```python
from build123d import *

# Parameters (mm, degrees)
F0_W     = 48.799998641
F0_H     = 16.799998641
F0_W_2   = 44.799998641
F0_H_2   = 12.799998641
F0_W_3   = 44
F0_H_3   = 12
F0_W_4   = 40
F0_H_4   = 8
F1_DEPTH = 13
F2_DEPTH = 10.5
F3_R     = 2
F4_R     = 2
F6_DEPTH = 25
F7_R     = 7.99999


# Not quite as in the source:
# - a fillet or chamfer is up to 0.001 mm smaller than in the source, because OpenCascade refuses the exact size


with BuildPart() as f1:
    # F0 (on Top) → F1 (new body)
    with BuildSketch(Plane.XY):
        Rectangle(F0_W, F0_H)
        Rectangle(F0_W_2, F0_H_2, mode=Mode.SUBTRACT)
        Rectangle(F0_W_2, F0_H_2)
        Rectangle(F0_W_3, F0_H_3, mode=Mode.SUBTRACT)
        Rectangle(F0_W_3, F0_H_3)
        Rectangle(F0_W_4, F0_H_4, mode=Mode.SUBTRACT)
        Rectangle(F0_W_4, F0_H_4)
    extrude(amount=F1_DEPTH)

    # F0 (on Top) → F2 (cut)
    with BuildSketch(Plane.XY):
        Rectangle(F0_W_2, F0_H_2)
        Rectangle(F0_W_3, F0_H_3, mode=Mode.SUBTRACT)
        Rectangle(F0_W_3, F0_H_3)
        Rectangle(F0_W_4, F0_H_4, mode=Mode.SUBTRACT)
        Rectangle(F0_W_4, F0_H_4)
    extrude(amount=F2_DEPTH, mode=Mode.SUBTRACT)

    # F3
    f3_edges = [f1.edges().sort_by_distance(p)[0] for p in [
        (-24.399999, -8.399999, 6.5),
        (-24.399999, 8.399999, 6.5),
        (24.399999, -8.399999, 6.5),
        (24.399999, 8.399999, 6.5),
    ]]
    fillet(f3_edges, radius=F3_R)

    # F4
    f4_edges = [f1.edges().sort_by_distance(p)[0] for p in [
        (-22.399999, -6.399999, 5.25),
        (22.399999, -6.399999, 5.25),
        (22.399999, 6.399999, 5.25),
        (-22.399999, 6.399999, 5.25),
    ]]
    fillet(f4_edges, radius=F4_R)

    # F5 (on face) → F6 (join)
    with BuildSketch(Plane(origin=(0, 0, 0), x_dir=(1, 0, 0), z_dir=(0, 0, -1))):
        Polygon((-8, 6.3999993205), (0, 6.3999993205), (8, 6.3999993205), (8, 8.3999993205), (-8, 8.3999993205), align=None)
        Polygon((8, -8.3999993205), (8, -6.3999993205), (0, -6.3999993205), (-8, -6.3999993205), (-8, -8.3999993205), align=None)
    extrude(amount=F6_DEPTH)

    # F7 (radius 8 in the source; OpenCascade refuses exactly that, so slightly less here)
    f7_edges = [f1.edges().sort_by_distance(p)[0] for p in [
        (-8, -7.399999, -25),
        (8, -7.399999, -25),
        (-8, 7.399999, -25),
        (8, 7.399999, -25),
    ]]
    fillet(f7_edges, radius=F7_R)


solid = f1.part
```
Geometry: final body of the model. Coordinates: model frame, mm. A direction names the side the tool comes from. Round coordinates to 2 decimals unless told otherwise and drop trailing zeros. Order: outer loops, then holes, each group sorted by start corner. A loop starts at its lowest first (then second) coordinate and runs counter-clockwise, first axis right, second up. Notation, with made-up numbers: (16, 68.5) -> (65, 68.5) arc R23 cw to (65, 100.5) -> close; hole circle Ø10 at (7.25, 40.5). An arc over 180 degrees is marked (long way). Use CSV: the item, a comma, the result in double quotes. Start each with the question number.
1) First-contact query: pin 1 Ø1 at (x, y) = (9, 2.5) entering from -Z; pin 2 Ø1 at (y, z) = (7, -8.5) entering from -X; pin 3 Ø1 at (y, z) = (7.5, -12.5) entering from +X. Flat tips, straight axial feed; report the tip coordinate or a pass-through.
2) Section A-A (z = 7.5). Return the cut outline in (x, y), and give its area (3 significant figures).
3) Section D-D (y = 3). Return the cut outline in (x, z).
4) Set-up query: faces 1 (the face through (-8, 7, -8)), 2 (the face through (21.83, 5.8, 5.32)), 3 (the face through (-24.4, 0, 6)). Return all of +Z, -Z, +X, -X, +Y, -Y with unobstructed straight access to the full face (end or side cutting, diameter ignored); none if empty.
5) Draft query along Y for faces 4 (the face through (-21.8, -5.83, 5.32)), 5 (the face through (23.8, 7.83, 6.59)), 6 (the face through (8, 7, -8)), 7 (the face through (0, 0, 10.5)). Return one class per face: +Y half, -Y half, draft (parallel to the pull), parting line (faces both ways), or undercut.
6) Section C-C (z = -15.5). Return the cut outline in (x, y).
7) Material intervals for line 1 along Y through (x, z) = (-2, 9.5); line 2 along X through (y, z) = (-2.25, 1.5); line 3 along Z through (x, y) = (13, 4.25), sorted ascending. Write a range as from..to.
8) Section B-B (x = 10.5). Return the cut outline in (y, z).
Returned:
1,pin 1,"stops at z = 10.5"
1,pin 2,"stops at x = -8"
1,pin 3,"stops at x = 8"
2,outline,"(-24.4, -6.4) arc R2 ccw to (-22.4, -8.4) -> (22.4, -8.4) arc R2 ccw to (24.4, -6.4) -> (24.4, 6.4) arc R2 ccw to (22.4, 8.4) -> (-22.4, 8.4) arc R2 ccw to (-24.4, 6.4) -> close; hole (-22.4, -4.4) arc R2 ccw to (-20.4, -6.4) -> (20.4, -6.4) arc R2 ccw to (22.4, -4.4) -> (22.4, 4.4) arc R2 ccw to (20.4, 6.4) -> (-20.4, 6.4) arc R2 ccw to (-22.4, 4.4) -> close"
2,area,"246 mm²"
3,outline,"(-24.4, 0) -> (-22.4, 0) -> (-22.4, 10.5) -> (22.4, 10.5) -> (22.4, 0) -> (24.4, 0) -> (24.4, 13) -> (-24.4, 13) -> close"
4,face 1,"-Z, -X, +Y, -Y"
4,face 2,"-Z"
4,face 3,"+Z, -Z, -X, +Y, -Y"
5,face 4,"undercut"
5,face 5,"+Y half"
5,face 6,"draft"
5,face 7,"undercut"
6,outline,"(-8, -8.4) -> (8, -8.4) -> (8, -6.4) -> (-8, -6.4) -> close; (-8, 6.4) -> (8, 6.4) -> (8, 8.4) -> (-8, 8.4) -> close"
7,line 1,"y = -8.4..-6.4, 6.4..8.4"
7,line 2,"x = -24.4..-22.4, 22.4..24.4"
7,line 3,"z = 10.5..13"
8,outline,"(-8.4, 0) -> (-6.4, 0) -> (-6.4, 10.5) -> (6.4, 10.5) -> (6.4, 0) -> (8.4, 0) -> (8.4, 13) -> (-8.4, 13) -> close"
